from build123d import *

# Parameters (mm, degrees)
F0_W      = 10
F0_H      = 50
F0_H_2    = 9.678417
F1_DEPTH  = 4
F2_DEPTH  = 5
F4_DEPTH  = 10
F5_DEPTH  = 5
F6_DEPTH  = 10
F7_DEPTH  = 4
F9_DEPTH  = 10
F10_DEPTH = 10
F11_DEPTH = 10
F8_W      = 2
F8_H      = 2.450932
F8_W_2    = 3
F12_DEPTH = 10


with BuildPart() as f1:
    # F0 (on Right) → F1 (new body)
    with BuildSketch(Plane.YZ):
        with BuildLine():
            ThreePointArc((0, 0), (22.928417, 22.928417), (0, 45.856834))
            Line((0, 45.856834), (0, 36.178417))
            ThreePointArc((0, 36.178417), (13.25, 22.928417), (0, 9.678417))
            Line((0, 9.678417), (0, 0))
        make_face()
        with Locations((-5, -25)):
            Rectangle(F0_W, F0_H)
        with Locations((-5, 4.839208)):
            Rectangle(F0_W, F0_H_2)
        with Locations((-5, 41.017625)):
            Rectangle(F0_W, F0_H_2)
        with Locations((-5, 70.856834)):
            Rectangle(F0_W, F0_H)
    extrude(amount=F1_DEPTH)

    # F0 (on Right) → F2 (join)
    with BuildSketch(Plane.YZ):
        with Locations((-5, 70.856834)):
            Rectangle(F0_W, F0_H)
        with Locations((-5, -25)):
            Rectangle(F0_W, F0_H)
        with BuildLine():
            ThreePointArc((0, 0), (22.928417, 22.928417), (0, 45.856834))
            Line((0, 45.856834), (0, 36.178417))
            ThreePointArc((0, 36.178417), (13.25, 22.928417), (0, 9.678417))
            Line((0, 9.678417), (0, 0))
        make_face()
    extrude(amount=F2_DEPTH)

    # F3 (on Front) → F4 (join, through all)
    with BuildSketch(Plane.XZ):
        with BuildLine():
            Line((-7.4979, -57.686251), (-2.503859, -57.686251))
            ThreePointArc((-2.503859, -57.686251), (2.489394, -52.692998), (7.482647, -57.686251))
            Line((7.482647, -57.686251), (12.501129, -57.686251))
            ThreePointArc((12.501129, -57.686251), (10.28152, -52.251641), (4.882479, -49.946863))
            Line((4.882479, -49.946863), (0, -49.946863))
            ThreePointArc((0, -49.946863), (-5.336135, -52.278896), (-7.4979, -57.686251))
        make_face()
        with BuildLine():
            Line((12.500054, 103.57853), (7.508172, 103.57853))
            ThreePointArc((7.508172, 103.57853), (2.492773, 98.583596), (-2.522626, 103.57853))
            Line((-2.522626, 103.57853), (-7.575432, 103.57853))
            ThreePointArc((-7.575432, 103.57853), (-5.361949, 98.175121), (0, 95.863014))
            Line((0, 95.863014), (5.021239, 95.826961))
            ThreePointArc((5.021239, 95.826961), (10.295439, 98.221958), (12.500054, 103.57853))
        make_face()
        with BuildLine():
            ThreePointArc((-2.522626, 103.57853), (2.492773, 108.59393), (7.508172, 103.57853))
            Line((7.508172, 103.57853), (12.500054, 103.57853))
            ThreePointArc((12.500054, 103.57853), (2.462311, 113.635186), (-7.575432, 103.57853))
            Line((-7.575432, 103.57853), (-2.522626, 103.57853))
        make_face()
    extrude(amount=F4_DEPTH)

    # F0 (on Right) → F5 (join)
    with BuildSketch(Plane.YZ):
        with Locations((-5, 4.839208)):
            Rectangle(F0_W, F0_H_2)
        with BuildLine():
            ThreePointArc((0, 0), (22.928417, 22.928417), (0, 45.856834))
            Line((0, 45.856834), (0, 36.178417))
            ThreePointArc((0, 36.178417), (13.25, 22.928417), (0, 9.678417))
            Line((0, 9.678417), (0, 0))
        make_face()
        with Locations((-5, 41.017625)):
            Rectangle(F0_W, F0_H_2)
        with Locations((-5, 70.856834)):
            Rectangle(F0_W, F0_H)
        with Locations((-5, -25)):
            Rectangle(F0_W, F0_H)
    extrude(amount=F5_DEPTH)

    # F3 (on Front) → F6 (join)
    with BuildSketch(Plane.XZ):
        with BuildLine():
            ThreePointArc((7.482647, -57.686251), (2.489394, -62.699619), (-2.503859, -57.686251))
            Line((-2.503859, -57.686251), (-7.4979, -57.686251))
            ThreePointArc((-7.4979, -57.686251), (2.501614, -67.627111), (12.501129, -57.686251))
            Line((12.501129, -57.686251), (7.482647, -57.686251))
        make_face()
    extrude(amount=F6_DEPTH)

    # F0 (on Right) → F7 (join)
    with BuildSketch(Plane.YZ):
        with BuildLine():
            ThreePointArc((0, 0), (22.928417, 22.928417), (0, 45.856834))
            Line((0, 45.856834), (0, 36.178417))
            ThreePointArc((0, 36.178417), (13.25, 22.928417), (0, 9.678417))
            Line((0, 9.678417), (0, 0))
        make_face()
        with Locations((-5, 4.839208)):
            Rectangle(F0_W, F0_H_2)
        with Locations((-5, 41.017625)):
            Rectangle(F0_W, F0_H_2)
    extrude(amount=F7_DEPTH)

    # F8 (on face) → F9 (join, through all)
    with BuildSketch(Plane.XZ.offset(10)):
        with BuildLine():
            Line((7, -2.450932), (5, -2.450932))
            Line((5, -2.450932), (5, -49.949365))
            ThreePointArc((5, -49.949365), (6.010656, -50.045316), (7, -50.272981))
            Line((7, -50.272981), (7, -49.946863))
            Line((7, -49.946863), (7, -2.450932))
        make_face()
    extrude(amount=-F9_DEPTH)

    # F8 (on face) → F10 (join, through all)
    with BuildSketch(Plane.XZ.offset(10)):
        with BuildLine():
            Line((0, -2.450932), (-3, -2.450932))
            Line((-3, -2.450932), (-3, -50.632482))
            ThreePointArc((-3, -50.632482), (-1.534725, -50.137731), (0, -49.946863))
            Line((0, -49.946863), (0, -2.450932))
        make_face()
    extrude(amount=-F10_DEPTH)

    # F8 (on face) → F11 (join, through all)
    with BuildSketch(Plane.XZ.offset(10)):
        Polygon((7, 46.067663), (7, 63.85126), (7, 95.866434), (7, 96.559308), (-3, 96.559308), (-3, 95.866434), (-3, 63.85126), (-3, 46.438996), (-2.991397, 45.816407), (0, 45.816407), (3.942358, 45.816407), (7, 45.816407), align=None)
    extrude(amount=-F11_DEPTH)

    # F8 (on face) → F12 (join, through all)
    with BuildSketch(Plane.XZ.offset(10)):
        with Locations((6, -1.225466)):
            Rectangle(F8_W, F8_H)
        with Locations((-1.5, -1.225466)):
            Rectangle(F8_W_2, F8_H)
    extrude(amount=-F12_DEPTH)


solid = f1.part
Verification items for the finished model (mm, model axes). A direction names the side the tool comes from. Give positions to 0.01 mm unless a question says otherwise; leave off trailing zeros. Loops run counter-clockwise (first coordinate to the right, second up) from the corner with the lowest first, then second, coordinate; pieces in that order, holes last. Notation, with made-up numbers: (43.5, -29.5) - (100.5, -29.5) arc R21 ccw to (100.5, -3.5) - close; hole circle Ø9 at (52.25, 1.25). An arc over 180 degrees is marked (long way). Write item = value, one per line. Start each with the question number.
Q1. Mould release check, pull along X, two halves, no side actions. Record for faces 1 (the face through (2.382, -4.93, 108.593)), 2 (the face through (7, -5, -25)), 3 (the face through (-3, -5, -25)): released by +X, released by -X, zero draft, split by the parting line, or undercut.
Q2. Cross-section at B-B, the plane z = -35.5. Enter the section's corners in (x, y), and give its area (3 significant figures).
Q3. Cross-section at C-C, the plane x = -4.75. Enter the section's corners in (y, z), and give its area (3 significant figures).
Q4. Cross-section at D-D, the plane y = 16. Enter the section's corners in (x, z).
Q5. Tool access check on faces 4 (the face through (2, 0, 80)), 5 (the face through (7, -5, 71)), 6 (the face through (2.6, -4.9, -62.7)), 7 (the face through (-3, -5, 72)). Record the directions out of +Z, -Z, +X, -X, +Y, -Y that give a thin tool (end or side, any length) a straight path to the whole face; none if there is none.
Q6. Cross-section at A-A, the plane x = 2.25. Enter the section's corners in (y, z), and give its area (3 significant figures).
Q7. Depth check by flat-ended pin: P1, Ø12, axis at y = 2.5, z = 68.5, coming from the -X side; P2, Ø16.5, axis at y = 11, z = 27, coming from the +X side; P3, Ø2.5, axis at x = -2, y = -5.5, coming from the -Z side; P4, Ø1.5, axis at x = 3, y = -7, coming from the +Z side. Enter the tip coordinate at first touch or a pass-through.
Q8. Thickness scan on line 1 (Z direction, x = 4.25, y = -2.5); line 2 (Y direction, x = -0.75, z = -27); line 3 (Z direction, x = 3.5, y = 10.5). Record the ranges inside material, lowest first.
Answer key:
q1.face_1 = undercut
q1.face_2 = released by +X
q1.face_3 = released by -X
q2.outline = (-3, -10) - (7, -10) - (7, 0) - (-3, 0) - close
q2.area = 100 mm^2
q3.outline = (-10, -64.51) - (0, -64.51) - (0, -51.73) - (-10, -51.73) - close; (-10, 97.62) - (0, 97.62) - (0, 110.58) - (-10, 110.58) - close
q3.area = 257 mm^2
q4.outline = (0, 6.51) - (5, 6.51) - (5, 39.35) - (0, 39.35) - close
q5.face_4 = +Z, +X, -X, +Y
q5.face_5 = +X, +Y, -Y
q5.face_6 = +Y, -Y
q5.face_7 = -X, +Y, -Y
q6.outline = (-10, -67.62) - (0, -67.62) - (0, -62.69) - (-10, -62.69) - close; (-10, -52.7) - (0, -52.7) - (0, 0) arc R22.93 ccw to (0, 45.86) - (0, 98.59) - (-10, 98.59) - (-10, 36.18) - (0, 36.18) arc R13.25 cw to (0, 9.68) - (-10, 9.68) - close; (-10, 108.59) - (0, 108.59) - (0, 113.63) - (-10, 113.63) - close
q6.area = 1,900 mm^2
q7.P1 = -3
q7.P2 = 5
q7.P3 = -67.08
q7.P4 = 113.64
q8.line_1 = -67.47 to -62.38, -53.01 to 9.68, 36.18 to 98.9, 108.28 to 113.47
q8.line_2 = -10 to 0
q8.line_3 = 2.55 to 14.85, 31.01 to 43.31
